from build123d import *

# Parameters (mm, degrees)
CROQUIS2_R              = 2.5
SALIENTE_EXTRUIR1_DEPTH = 4


with BuildPart() as part:
    # Croquis2 → Saliente-Extruir1 (new body)
    with BuildSketch(Plane(origin=(0, 0, 0), x_dir=(1, 0, 0), z_dir=(0, 1, 0))):
        with BuildLine():
            Line((-79.601178676, 51.546233526), (-16.651724566, 61.929211291))
            Line((-16.651724566, 61.929211291), (-16.651724566, -24.070788709))
            Line((-16.651724566, -24.070788709), (-79.565967679, -13.476544348))
            add(Edge.make_bspline(
                [(-79.601178676, 51.546233526), (-91.719874733, 19.028313012), (-79.565967679, -13.476544348)],
                knots=[0, 0, 0, 1, 1, 1], degree=2))
        make_face()
        with Locations((-81.212594438, 19.032720929)):
            Circle(CROQUIS2_R, mode=Mode.SUBTRACT)
    extrude(amount=SALIENTE_EXTRUIR1_DEPTH)


solid = part.part
Work out the finished part from the listing and answer in its coordinate system (mm). Round coordinates to 2 decimals unless told otherwise and drop trailing zeros. Order: outer loops, then holes, each group sorted by start corner. A loop starts at its lowest first (then second) coordinate and runs counter-clockwise, first axis right, second up. Notation, with made-up numbers: M 62,36 L 86,36 A22 cw 86,69 Z; hole C 77,-18.75 d10. An arc over 180 degrees is marked long. One line per item, written item: value.
Q1. Flat-ended cylindrical pins translate along their axes: pin 1 (1 mm diameter, centred on y = 1.5, z = -13, fed in from -X); pin 2 (2 mm diameter, centred on y = 2, z = -2.5, fed in from -X). Find the tip coordinate at first contact, or state that the pin passes through.
Derived:
pin 1: x = -85.47
pin 2: x = -84.26
Q2. Straight lines are drawn through the part: line 1 (X direction, y = 3.3, z = -51.5); line 2 (X direction, y = 1.8, z = -23.5); line 3 (Z direction, x = -19.5, y = 1.45). For each, find the intervals that lie inside material, in ascending order.
Derived:
line 1: -79.62 to -16.65
line 2: -85.54 to -16.65
line 3: -61.46 to 23.59
Q3. Find section A-A on x = -49.5. Write down the section's boundary in (y, z), then the cut area to 3 significant figures.
Derived:
outline: M 0,-56.51 L 4,-56.51 L 4,18.54 L 0,18.54 Z
area: 300 mm²
Q4. Find section B-B on x = -34.5. Write down the section's boundary in (y, z), then the cut area to 3 significant figures.
Derived:
outline: M 0,-58.99 L 4,-58.99 L 4,21.07 L 0,21.07 Z
area: 320 mm²
